Part model, mm, in its own coordinate system. A direction names the side the tool comes from. Coordinates: 2 decimals unless noted, no trailing zeros. Loops run counter-clockwise (first coordinate to the right, second up) from the corner with the lowest first, then second, coordinate; pieces in that order, holes last. Notation, with made-up numbers: M -32.75,-2.5 L -5.75,-2.5 A12 cw -5.75,7.5 Z; hole C -34.5,-28.5 d9. An arc over 180 degrees is marked long. Use a Markdown table: item, result. Add a question column.
1) Pin check, flat tips, straight feed: pin 1 Ø4.5 at (x, y) = (6.91, -64) entering from +Z; pin 2 Ø7 at (x, y) = (-33.09, 9) entering from +Z. Stop position of each tip, or through.
2) Band-saw the part on A-A (y = -77). List the corners of the cut face in (x, z), plus the area to 3 significant figures.
3) Wall check: probe 1 along X at (y, z) = (9, -7.25); probe 2 along Y at (x, z) = (5, -5.75); probe 3 along X at (y, z) = (-77, -7.5). Give the ranges that are in metal, low to high. Write a range as from..to.
4) Band-saw the part on B-B (z = -3.25). List the corners of the cut face in (x, y), plus the area to 3 significant figures.
5) Band-saw the part on D-D (y = -16). List the corners of the cut face in (x, z).
6) Band-saw the part on C-C (y = 9). List the corners of the cut face in (x, z).
7) Tool access for faces 5 (the flat face through (-13, -41, -7.963)), 6 (the conical face through (-32.68, 12.18, -5.11)): list every direction of +Z, -Z, +X, -X, +Y, -Y with a clear straight run to the whole face (end or side of a thin tool).
8) Pull direction Z, two halves, no side cores. Call faces 1 (the flat face through (-5.642, -41.412, -4.414)), 2 (the conical face through (-32.4, -80.13, -5.11)), 3 (the conical face through (9.27, -66.17, -8.82)), 4 (the cylindrical face through (-32.735, -74.273, -9.481)): released by +Z, released by -Z, zero draft, split by the parting line, or undercut.
from build123d import *

# Parameters (mm, degrees)
F1_DEPTH       = 84
F2_DEPTH       = 16
F4_D           = 5.5
F4_CSINK_D     = 11.2
F4_CSINK_ANGLE = 60
F6_D           = 5.5
F6_CSINK_D     = 11.2
F6_CSINK_ANGLE = 60


with BuildPart() as f1:
    # F0 (on Front) → F1 (new body)
    with BuildSketch(Plane.XZ):
        Polygon((-48.092596, -0.963417), (-48.092596, -12.963417), (21.907404, -12.963417), (21.907404, -0.963417), (-7.634048, -0.963417), (-3.592596, -7.963417), (-13.092596, -7.963417), (-22.592596, -7.963417), (-18.551144, -0.963417), align=None)
    extrude(amount=F1_DEPTH)

    # F0 (on Front) → F2 (join)
    with BuildSketch(Plane.XZ):
        Polygon((-48.092596, -0.963417), (-48.092596, -12.963417), (21.907404, -12.963417), (21.907404, -0.963417), (-7.634048, -0.963417), (-3.592596, -7.963417), (-13.092596, -7.963417), (-22.592596, -7.963417), (-18.551144, -0.963417), align=None)
        Polygon((-7.634048, -0.963417), (-18.551144, -0.963417), (-22.592596, -7.963417), (-13.092596, -7.963417), (-3.592596, -7.963417), align=None)
    extrude(amount=-F2_DEPTH)

    # F4 (through all)
    with Locations(Plane.XY.offset(-0.963417)):
        with Locations((-33.092596, 9), (6.907404, 9), (6.907404, -77), (-33.092596, -77)):
            CounterSinkHole(F4_D / 2, F4_CSINK_D / 2, counter_sink_angle=F4_CSINK_ANGLE)

    # F6 (through all)
    with Locations(Plane(origin=(0, 0, -12.963417), x_dir=(1, 0, 0), z_dir=(0, 0, -1))):
        with Locations((-33.092596, 64), (6.907404, 64)):
            CounterSinkHole(F6_D / 2, F6_CSINK_D / 2, counter_sink_angle=F6_CSINK_ANGLE)


solid = f1.part
Entries:
| question | item | result |
|---|---|---|
| 1 | pin 1 | through |
| 1 | pin 2 | z = -4.6 |
| 2 | outline | M -48.09,-12.96 L -35.84,-12.96 L -35.84,-5.9 L -38.69,-0.96 L -48.09,-0.96 Z; M -30.34,-12.96 L 4.16,-12.96 L 4.16,-5.9 L 1.31,-0.96 L -7.63,-0.96 L -3.59,-7.96 L -22.59,-7.96 L -18.55,-0.96 L -27.49,-0.96 L -30.34,-5.9 Z; M 9.66,-12.96 L 21.91,-12.96 L 21.91,-0.96 L 12.51,-0.96 L 9.66,-5.9 Z |
| 2 | area | 575 mm2 |
| 3 | probe 1 | -48.09..-35.84, -30.34..4.16, 9.66..21.91 |
| 3 | probe 2 | -84..-79.1, -74.9..-65.98, -62.02..6.9, 11.1..16 |
| 3 | probe 3 | -48.09..-35.84, -30.34..-22.33, -3.86..4.16, 9.66..21.91 |
| 4 | outline | M -48.09,-84 L -19.87,-84 L -19.87,0 L -6.31,0 L -6.31,-84 L 21.91,-84 L 21.91,16 L -48.09,16 Z; hole C -33.09,-77 d8.56; hole C -33.09,9 d8.56; hole C -33.09,-64 d5.5; hole C 6.91,-77 d8.56; hole C 6.91,9 d8.56; hole C 6.91,-64 d5.5 |
| 4 | area | 5,580 mm2 |
| 5 | outline | M -48.09,-12.96 L 21.91,-12.96 L 21.91,-0.96 L -7.63,-0.96 L -3.59,-7.96 L -22.59,-7.96 L -18.55,-0.96 L -48.09,-0.96 Z |
| 6 | outline | M -48.09,-12.96 L -35.84,-12.96 L -35.84,-5.9 L -38.69,-0.96 L -48.09,-0.96 Z; M -30.34,-12.96 L 4.16,-12.96 L 4.16,-5.9 L 1.31,-0.96 L -27.49,-0.96 L -30.34,-5.9 Z; M 9.66,-12.96 L 21.91,-12.96 L 21.91,-0.96 L 12.51,-0.96 L 9.66,-5.9 Z |
| 7 | face 5 | -Y |
| 7 | face 6 | +Z |
| 8 | face 1 | undercut |
| 8 | face 2 | released by +Z |
| 8 | face 3 | released by -Z |
| 8 | face 4 | zero draft |
